```python
from build123d import *

# Parameters (mm, degrees)
SKETCH1_R           = 7
BOSS_EXTRUDE1_DEPTH = 8
CUT_EXTRUDE4_START  = -42.686292
CUT_EXTRUDE4_DEPTH  = 192


with BuildPart() as part:
    # Sketch1 → Boss-Extrude1 (new body)
    with BuildSketch(Plane(origin=(0, 0, 0), x_dir=(1, 0, 0), z_dir=(0, 1, 0))):
        Polygon((0, -21.713615023), (54, 32.286384977), (11.313708499, 32.286384977), (-42.686291501, 32.286384977), (-42.686291501, -21.713615023), align=None)
        with Locations((-15.686291501, 5.286384977)):
            Circle(SKETCH1_R, mode=Mode.SUBTRACT)
    extrude(amount=BOSS_EXTRUDE1_DEPTH)

    # Sketch4 → Cut-Extrude4 (cut)
    with BuildSketch(Plane(origin=(0, 0, 0), x_dir=(0, 0, -1), z_dir=(1, 0, 0)).offset(CUT_EXTRUDE4_START)):
        Polygon((32.286384977, 0), (24.286384977, 8), (32.286384977, 8), align=None)
    extrude(amount=CUT_EXTRUDE4_DEPTH, mode=Mode.SUBTRACT)


solid = part.part
```
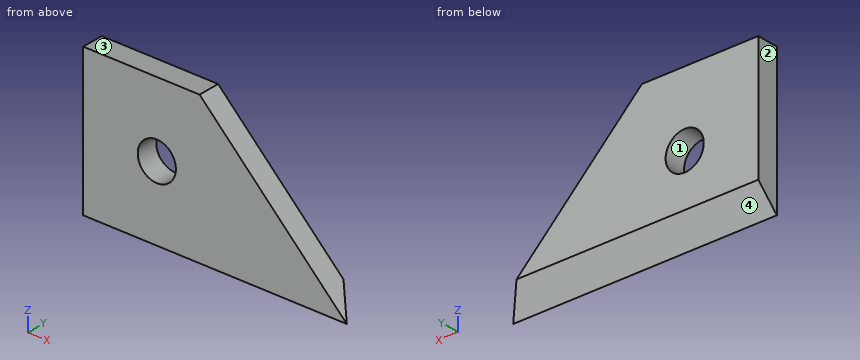
Verification items for the finished model (mm, model axes). Face numbers are marked on the shaded views. Give positions to 0.01 mm unless a question says otherwise; leave off trailing zeros. Write each loop counter-clockwise with the first axis right and the second up, starting at its lowest first coordinate (ties: lowest second). Pieces come first, ordered by that corner, then holes. Notation, with made-up numbers: (39.5, 74.25) - (72.5, 74.25) arc R20 ccw to (72.5, 79.25) - close; hole circle Ø10 at (15.25, 85.5). An arc over 180 degrees is marked (long way). Put each result on its own line as item: value.
Q1. Section check A-A on x = -12. Record the cut outline in (y, z).
Result:
outline: (0, -32.29) - (8, -24.29) - (8, -11.24) - (0, -11.24) - close; (0, 0.66) - (8, 0.66) - (8, 21.71) - (0, 21.71) - close
Q2. Depth check by flat-ended pin: P1, Ø2, axis at y = 3.5, z = -7.5, coming from the +X side; P2, Ø2, axis at x = 19.5, y = 2, coming from the +Z side. Enter the tip coordinate at first touch or a pass-through.
Result:
P1: x = 30.21
P2: z = 3.21
Q3. Mould release check, pull along Z, two halves, no side actions. Record for the marked faces 1, 2, 3 and 4: released by +Z, released by -Z, zero draft, split by the parting line, or undercut.
Result:
face 1: undercut
face 2: zero draft
face 3: released by +Z
face 4: released by -Z
Q4. Section check B-B on y = 5.5. Record the cut outline in (x, z), and give its area (3 significant figures).
Result:
outline: (-42.69, -26.79) - (48.5, -26.79) - (0, 21.71) - (-42.69, 21.71) - close; hole circle Ø14 at (-15.69, -5.29)
area: 3,090 mm2
Q5. Section check C-C on z = -22. Record the cut outline in (x, y).
Result:
outline: (-42.69, 0) - (43.71, 0) - (43.71, 8) - (-42.69, 8) - close
Q6. Scan lines: probe 1 along X at (y, z) = (6, -7.5); probe 2 along X at (y, z) = (3, -8); probe 3 along Z at (x, y) = (-18, 3.75). Record each from-to range of solid material in increasing order. Write a range as from..to.
Result:
probe 1: -42.69..-22.33, -9.05..29.21
probe 2: -42.69..-22.14, -9.23..29.71
probe 3: -28.54..-11.89, 1.32..21.71
Q7. Section check D-D on x = 8.5. Record the cut outline in (y, z), and give its area (3 significant figures).
Result:
outline: (0, -32.29) - (8, -24.29) - (8, 13.21) - (0, 13.21) - close
area: 332 mm2
